from build123d import *

# Parameters (mm, degrees)
BOSS_EXTRUDE1_DEPTH = 40
SKETCH2_R           = 1.5
CUT_EXTRUDE1_DEPTH  = 7.1
CUT_EXTRUDE3_DEPTH  = 3


with BuildPart() as part:
    # Sketch1 → Boss-Extrude1 (new body)
    with BuildSketch(Plane.XY):
        Polygon((-2.460653528, 0), (2.460653528, 0), (5.25, 2.789346472), (5.25, 4.3), (3.065, 4.3), (4.865, 6.1), (-4.865, 6.1), (-3.065, 4.3), (-5.25, 4.3), (-5.25, 2.789346472), align=None)
    extrude(amount=BOSS_EXTRUDE1_DEPTH)

    # Sketch2 → Cut-Extrude1 (cut, through all)
    with BuildSketch(Plane(origin=(0, 6.1, 0), x_dir=(1, 0, 0), z_dir=(0, 1, 0))):
        with Locations((0, -30)):
            Circle(SKETCH2_R)
        with Locations((0, -10)):
            Circle(SKETCH2_R)
    extrude(amount=-CUT_EXTRUDE1_DEPTH, mode=Mode.SUBTRACT)

    # Sketch5 → Cut-Extrude3 (cut)
    with BuildSketch(Plane(origin=(0, 0, 0), x_dir=(-1, 0, 0), z_dir=(0, -1, 0))):
        Polygon((-3.233161507, -10), (-1.616580754, -12.8), (1.616580754, -12.8), (3.233161507, -10), (1.616580754, -7.2), (-1.616580754, -7.2), align=None)
        Polygon((-3.233161507, -30), (-1.616580754, -32.8), (1.616580754, -32.8), (3.233161507, -30), (1.616580754, -27.2), (-1.616580754, -27.2), align=None)
    extrude(amount=-CUT_EXTRUDE3_DEPTH, mode=Mode.SUBTRACT)


solid = part.part
Here's how the part is built. I have some questions about the finished solid (model axes, mm). A direction names the side the tool comes from. Coordinates: 2 decimals unless noted, no trailing zeros. Loops run counter-clockwise (first coordinate to the right, second up) from the corner with the lowest first, then second, coordinate; pieces in that order, holes last.
1. I need wall thicknesses on L1, parallel to Z at x = 0, y = 5.15; L2, parallel to X at y = 3.85, z = 30; L3, parallel to Z at x = -0.5, y = 1.5. Which ranges of each line are inside material? Lowest first, please.
2. Imagine slicing it at D-D, the plane y = 2. Please give me the cut outline in (x, z), and give its area (3 significant figures).
3. For P1, Ø5, axis at x = 0, z = 30, coming from the -Y side, with a flat end and sliding along its axis, tell me the tip position at first contact or that it passes through.
4. For faces 5 (the flat face through (0, 1, 7.2)), 6 (the flat face through (0, 0, 37)), which set-ups out of +Z, -Z, +X, -X, +Y, -Y let a thin tool reach every point of the face, with its end or its side?
5. If we mould it in two halves opening along X, with no side actions, what happens to faces 1 (the flat face through (-2.436, 1.479, 28.62)), 2 (the flat face through (0, 0, 20)), 3 (the flat face through (3.84, 1.38, 19.72)), 4 (the flat face through (-3.87, 1.41, 19.72))? For each: pulls with the +X half, pulls with the -X half, needs draft (parallel to the pull), parting line crosses it, or undercut.
6. Imagine slicing it at A-A, the plane x = 0. Please give me the cut outline in (y, z).
7. Imagine slicing it at B-B, the plane z = 22.5. Please give me the cut outline in (x, y) (3 decimals), and give its area (3 significant figures).
8. Imagine slicing it at C-C, the plane z = 31. Please give me the cut outline in (x, y) (3 decimals), and give its area (3 significant figures).
Taken from the geometry:
1. L1: z = 0 to 8.5, 11.5 to 28.5, 31.5 to 40
1. L2: x = -5.25 to -1.5, 1.5 to 5.25
1. L3: z = 0 to 7.2, 12.8 to 27.2, 32.8 to 40
2. outline: (-4.46, 0) - (4.46, 0) - (4.46, 40) - (-4.46, 40) - close; hole (-3.23, 10) - (-1.62, 7.2) - (1.62, 7.2) - (3.23, 10) - (1.62, 12.8) - (-1.62, 12.8) - close; hole (-3.23, 30) - (-1.62, 27.2) - (1.62, 27.2) - (3.23, 30) - (1.62, 32.8) - (-1.62, 32.8) - close
2. area: 303 mm2
3. P1: stops at y = 3
4. face 5: -Y
4. face 6: +Z, -Z, +X, -X, -Y
5. face 1: undercut
5. face 2: needs draft
5. face 3: pulls with the +X half
5. face 4: pulls with the -X half
6. outline: (0, 0) - (6.1, 0) - (6.1, 8.5) - (3, 8.5) - (3, 7.2) - (0, 7.2) - close; (0, 12.8) - (3, 12.8) - (3, 11.5) - (6.1, 11.5) - (6.1, 28.5) - (3, 28.5) - (3, 27.2) - (0, 27.2) - close; (0, 32.8) - (3, 32.8) - (3, 31.5) - (6.1, 31.5) - (6.1, 40) - (0, 40) - close
7. outline: (-5.25, 2.789) - (-2.461, 0) - (2.461, 0) - (5.25, 2.789) - (5.25, 4.3) - (3.065, 4.3) - (4.865, 6.1) - (-4.865, 6.1) - (-3.065, 4.3) - (-5.25, 4.3) - close
7. area: 51.6 mm2
8. outline: (-5.25, 2.789) - (-2.656, 0.195) - (-2.656, 3) - (-1.118, 3) - (-1.118, 6.1) - (-4.865, 6.1) - (-3.065, 4.3) - (-5.25, 4.3) - close; (1.118, 3) - (2.656, 3) - (2.656, 0.195) - (5.25, 2.789) - (5.25, 4.3) - (3.065, 4.3) - (4.865, 6.1) - (1.118, 6.1) - close
8. area: 28.8 mm2
